CAD build for the part. Positions are in the model's coordinates, mm. Give positions to 0.01 mm unless a question says otherwise; leave off trailing zeros. Loops run counter-clockwise (first coordinate to the right, second up) from the corner with the lowest first, then second, coordinate; pieces in that order, holes last.
```python
from build123d import *

# Parameters (mm, degrees)
SKETCH1_R           = 2
BOSS_EXTRUDE2_DEPTH = 1


with BuildPart() as part:
    # Sketch1 → Boss-Extrude2 (new body, symmetric)
    with BuildSketch(Plane.XY):
        with BuildLine():
            Line((-16, 4), (16, 4))
            ThreePointArc((16, 4), (20, 0), (16, -4))
            Line((16, -4), (-16, -4))
            ThreePointArc((-16, -4), (-20, 0), (-16, 4))
        make_face()
        with Locations((-16, 0)):
            Circle(SKETCH1_R, mode=Mode.SUBTRACT)
        with Locations((16, 0)):
            Circle(SKETCH1_R, mode=Mode.SUBTRACT)
    extrude(amount=BOSS_EXTRUDE2_DEPTH, both=True)


solid = part.part
```
1. Saw through at A-A, the plane y = 0. List the corners of the cut face in (x, z), and give its area (3 significant figures).
Responses:
outline: (-20, -1) - (-18, -1) - (-18, 1) - (-20, 1) - close; (-14, -1) - (14, -1) - (14, 1) - (-14, 1) - close; (18, -1) - (20, -1) - (20, 1) - (18, 1) - close
area: 64.0 mm2
2. Probe line 1 along Y through (x, z) = (-16, -0.1); line 2 along X through (y, z) = (-0.25, 0.1); line 3 along X through (y, z) = (1.25, 0.9). List the from-to ranges inside material, lowest first.
Responses:
line 1: y = -4 to -2, 2 to 4
line 2: x = -19.99 to -17.98, -14.02 to 14.02, 17.98 to 19.99
line 3: x = -19.8 to -17.56, -14.44 to 14.44, 17.56 to 19.8
3. Drop a flat-ended pin along its axis: pin 1 (2.5 mm diameter, centred on x = 16, y = 0, fed in from +Z). Give the stop position or say it passes through.
Responses:
pin 1: passes through
4. Saw through at D-D, the plane y = -2.5. List the corners of the cut face in (x, z), and give its area (3 significant figures).
Responses:
outline: (-19.12, -1) - (19.12, -1) - (19.12, 1) - (-19.12, 1) - close
area: 76.5 mm2
5. Saw through at B-B, the plane x = -16.5. List the corners of the cut face in (y, z), and give its area (3 significant figures).
Responses:
outline: (-3.97, -1) - (-1.94, -1) - (-1.94, 1) - (-3.97, 1) - close; (1.94, -1) - (3.97, -1) - (3.97, 1) - (1.94, 1) - close
area: 8.13 mm2
6. Pull direction X, two halves, no side cores. Call faces 1 (the face through (-20, 0, 0)), 2 (the face through (0, 0, 1)), 3 (the face through (-17.6, -1.2, 0)): released by +X, released by -X, zero draft, split by the parting line, or undercut.
Responses:
face 1: released by -X
face 2: zero draft
face 3: undercut
7. Saw through at C-C, the plane z = 0.35. List the corners of the cut face in (x, y), and give its area (3 significant figures).
Responses:
outline: (-16, -4) - (16, -4) arc R4 ccw to (16, 4) - (-16, 4) arc R4 ccw to start; hole circle Ø4 at (-16, 0); hole circle Ø4 at (16, 0)
area: 281 mm2
